from build123d import *

# Parameters (mm, degrees)
BOSS_EXTRU_1_DEPTH      = 2.400000114
ESQUISSE9_W             = 36.19999811
ESQUISSE9_H             = 2.400000114
BOSS_EXTRU_2_DEPTH      = 5.365243182
ESQUISSE14_R            = 7.502289609
ENL_V_MAT_EXTRU_1_DEPTH = 72.901671136
ENL_V_MAT_EXTRU_2_DEPTH = 72.901671136
ESQUISSE25_R            = 1.252758793
ENL_V_MAT_EXTRU_3_DEPTH = 72.901671136
ESQUISSE28_R            = 2.406964412
BOSS_EXTRU_3_DEPTH      = 2.9


with BuildPart() as part:
    # Esquisse4 → Boss.-Extru.1 (new body)
    with BuildSketch(Plane.XY.offset(2.400000114)):
        with BuildLine():
            Line((-20.100001246, -24.634756148), (-48.900358379, 4.499999806))
            Line((-48.900358379, 4.499999806), (-60.405611992, 4.499999806))
            ThreePointArc((-60.405611992, 4.499999806), (-65.300002694, -0.500000082), (-60.405611992, -5.49999997))
            Line((-60.405611992, -5.49999997), (-56.299999356, -5.49999997))
            Line((-56.299999356, -5.49999997), (-56.299999356, -24.634756148))
            Line((-56.299999356, -24.634756148), (-20.100001246, -24.634756148))
        make_face()
    extrude(amount=-BOSS_EXTRU_1_DEPTH)

    # Esquisse9 → Boss.-Extru.2 (add)
    with BuildSketch(Plane(origin=(0, -24.634756148, 0), x_dir=(-1, 0, 0), z_dir=(0, -1, 0))):
        with Locations((38.200000301, -1.200000057)):
            Rectangle(ESQUISSE9_W, ESQUISSE9_H)
    extrude(amount=BOSS_EXTRU_2_DEPTH)

    # Esquisse14 → Enlèv. mat.-Extru.1 (cut, through all)
    with BuildSketch(Plane.XY.offset(2.400000114)):
        with Locations((-43.700002134, -16.999939794)):
            Circle(ESQUISSE14_R)
    extrude(amount=-ENL_V_MAT_EXTRU_1_DEPTH, mode=Mode.SUBTRACT)

    # Esquisse19 → Enlèv. mat.-Extru.2 (cut, through all)
    with BuildSketch(Plane.XY.offset(2.400000114)):
        Polygon((-26.350000873, -28.503000736), (-25.724001229, -28.334999457), (-25.264998898, -27.875998989), (-25.096999481, -27.249999344), (-25.264998898, -26.6239997), (-25.724001229, -26.165001094), (-26.350000873, -25.998000056), (-26.976000518, -26.165001094), (-27.434999123, -26.6239997), (-27.602000162, -27.249999344), (-27.434999123, -27.875998989), (-26.976000518, -28.334999457), align=None)
    extrude(amount=-ENL_V_MAT_EXTRU_2_DEPTH, mode=Mode.SUBTRACT)

    # Esquisse25 → Enlèv. mat.-Extru.3 (cut, through all)
    with BuildSketch(Plane(origin=(0, 0, 0), x_dir=(-1, 0, 0), z_dir=(0, 0, -1))):
        with Locations((50.350001082, -27.250241944)):
            Circle(ESQUISSE25_R)
    extrude(amount=-ENL_V_MAT_EXTRU_3_DEPTH, mode=Mode.SUBTRACT)

    # Esquisse28 → Boss.-Extru.3 (add)
    with BuildSketch(Plane.XY.offset(2.400000114)):
        with Locations((-60.267728087, -0.4991006)):
            Circle(ESQUISSE28_R)
    extrude(amount=BOSS_EXTRU_3_DEPTH)


solid = part.part
Could you check a few things on this model? Use its own coordinates, in mm. A direction names the side the tool comes from. Give positions to 0.01 mm unless a question says otherwise; leave off trailing zeros. Order: outer loops, then holes, each group sorted by start corner. A loop starts at its lowest first (then second) coordinate and runs counter-clockwise, first axis right, second up. Notation, with made-up numbers: (-33, 5) - (-28, 5) arc R30 cw to (-28, 29) - close; hole circle Ø3 at (-22, -2.75). An arc over 180 degrees is marked (long way). One line per item, written item: value. Start each with the question number.
1. Thinking about a two-plate mould opening in Y: for faces 4 (the face through (-58, -5.5, 1)), 5 (the face through (-20.1, -27, 1)), 6 (the face through (-49.43, -26.4, 1.18)), which applies, +Y half, -Y half, draft (parallel to the pull), parting line (faces both ways), or undercut?
2. Imagine slicing it at A-A on y = -21. List the corners of the cut face in (x, z) for me, plus the area to 3 significant figures.
3. If I drill on probe 1 along X at (y, z) = (-27, 2.1); probe 2 along Z at (x, y) = (-39.5, -25); probe 3 along Y at (x, z) = (-40.5, 0.35), over which ranges is the centre line in solid material (lowest first)?
4. Imagine slicing it at C-C on x = -55.5. List the corners of the cut face in (y, z) for me.
5. Imagine slicing it at D-D on y = 0.5. List the corners of the cut face in (x, z) for me, plus the area to 3 significant figures.
6. For faces 1 (the face through (-56.3, -18, 1)), 2 (the face through (-65.3, -0.4, 1.2)), 3 (the face through (-57.97, 0.22, 3.83)), which set-ups out of +Z, -Z, +X, -X, +Y, -Y let a thin tool reach every point of the face, with its end or its side?
7. Imagine slicing it at B-B on x = -44.5. List the corners of the cut face in (y, z) for me.
8. For P1, Ø1, axis at y = -16.5, z = 1, coming from the +X side; P2, Ø17, axis at x = -41, y = -13, coming from the +Z side; P3, Ø12, axis at x = -43.7, y = -17, coming from the -Z side; P4, Ø1.2, axis at y = -16, z = 1.5, coming from the -X side, each with a flat end and sliding along its axis, tell me the tip position at first contact or that it passes through.
Values:
1. face 4: -Y half
1. face 5: draft
1. face 6: undercut
2. outline: (-56.3, 0) - (-50.05, 0) - (-50.05, 2.4) - (-56.3, 2.4) - close; (-37.35, 0) - (-23.69, 0) - (-23.69, 2.4) - (-37.35, 2.4) - close
2. area: 47.8 mm²
3. probe 1: -56.3 to -51.58, -49.12 to -27.54, -25.16 to -20.1
3. probe 2: 0 to 2.4
3. probe 3: -30 to -23.79, -10.21 to -4
4. outline: (-30, 0) - (4.5, 0) - (4.5, 2.4) - (-30, 2.4) - close
5. outline: (-65.2, 0) - (-44.95, 0) - (-44.95, 2.4) - (-58.08, 2.4) - (-58.08, 5.3) - (-62.46, 5.3) - (-62.46, 2.4) - (-65.2, 2.4) - close
5. area: 61.3 mm²
6. face 1: +Z, -Z, -X, -Y
6. face 2: +Z, -Z, -X
6. face 3: +Z
7. outline: (-30, 0) - (-24.46, 0) - (-24.46, 2.4) - (-30, 2.4) - close; (-9.54, 0) - (0.05, 0) - (0.05, 2.4) - (-9.54, 2.4) - close
8. P1: x = -27.65
8. P2: z = 2.4
8. P3: through
8. P4: x = -56.3
